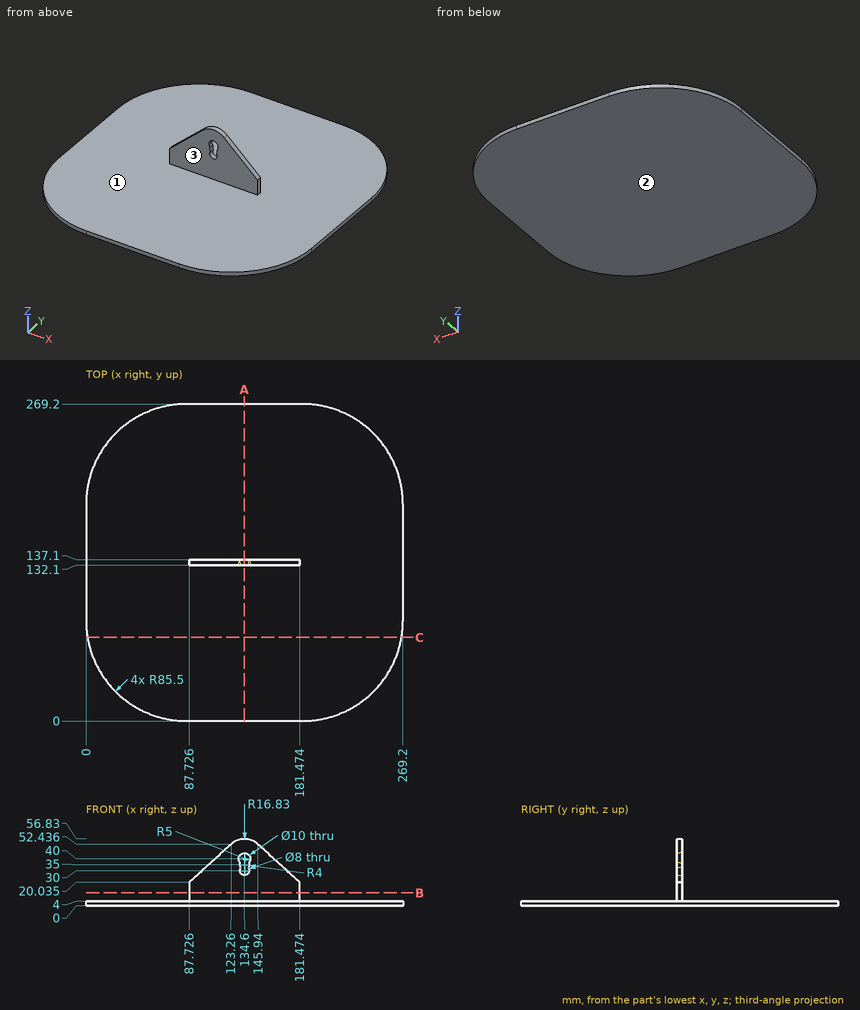
The drawing under review shows one solid part. Ordinate dimensions are in mm from its lowest x, y, z. Give positions to 0.01 mm unless a question says otherwise; leave off trailing zeros. Write each loop counter-clockwise with the first axis right and the second up, starting at its lowest first coordinate (ties: lowest second). Pieces come first, ordered by that corner, then holes. Notation, with made-up numbers: M 49.5,26 L 58.5,26 A27 ccw 58.5,42 Z; hole C 83.5,0.25 d2. An arc over 180 degrees is marked long. Write each question's results on one line, items separated by ' | '. Start each with the question number.
1. Mouldability with a two-part tool opening along Z and no side actions: class the marked faces 1, 2 and 3 as released by +Z, released by -Z, zero draft, split by the parting line, or undercut.
2. For probe 1 along Z at (x, y) = (134, 135) (1 decimal); probe 2 along Y at (x, z) = (155, 5); probe 3 along Z at (x, y) = (140.5, 81.5), list the stretches that pass through material, from the lowest coordinate up. Write a range as [from, to].
3. We need section A-A (x = 134.6). Write out the cut boundary in (y, z), and give its area (3 significant figures).
4. We need section C-C (y = 71). Write out the cut boundary in (x, z), and give its area (3 significant figures).
5. Insertion check: pin 1 Ø2.5 at (y, z) = (134.5, 10) entering from +X; pin 2 Ø6.5 at (x, z) = (134.6, 30) entering from +Y; pin 3 Ø4 at (y, z) = (135, 14.5) entering from -X; pin 4 Ø5 at (x, z) = (158.5, 32.5) entering from -Y. Each pin has a flat end and moves straight along its axis. Give the tip position at first contact, or say it passes through.
6. We need section B-B (z = 11). Write out the cut boundary in (x, y), and give its area (3 significant figures).
Results found:
1) face 1: released by +Z | face 2: released by -Z | face 3: zero draft
2) probe 1: z = [0, 26], [45, 56.8] | probe 2: y = [132.1, 137.1] | probe 3: z = [0, 4]
3) outline: M 0,0 L 269.2,0 L 269.2,4 L 137.1,4 L 137.1,26 L 132.1,26 L 132.1,4 L 0,4 Z; M 132.1,45 L 137.1,45 L 137.1,56.83 L 132.1,56.83 Z | area: 1,250 mm^2
4) outline: M 1.24,0 L 267.96,0 L 267.96,4 L 1.24,4 Z | area: 1,070 mm^2
5) pin 1: stops at x = 181.47 | pin 2: passes through | pin 3: stops at x = 87.73 | pin 4: stops at y = 132.1
6) outline: M 87.73,132.1 L 181.47,132.1 L 181.47,137.1 L 87.73,137.1 Z | area: 469 mm^2
